Here's the drawing with two shaded views (mm, measured from the low corner). I have some questions. A direction names the side the tool comes from. Coordinates: 2 decimals unless noted, no trailing zeros. Loops run counter-clockwise (first coordinate to the right, second up) from the corner with the lowest first, then second, coordinate; pieces in that order, holes last.
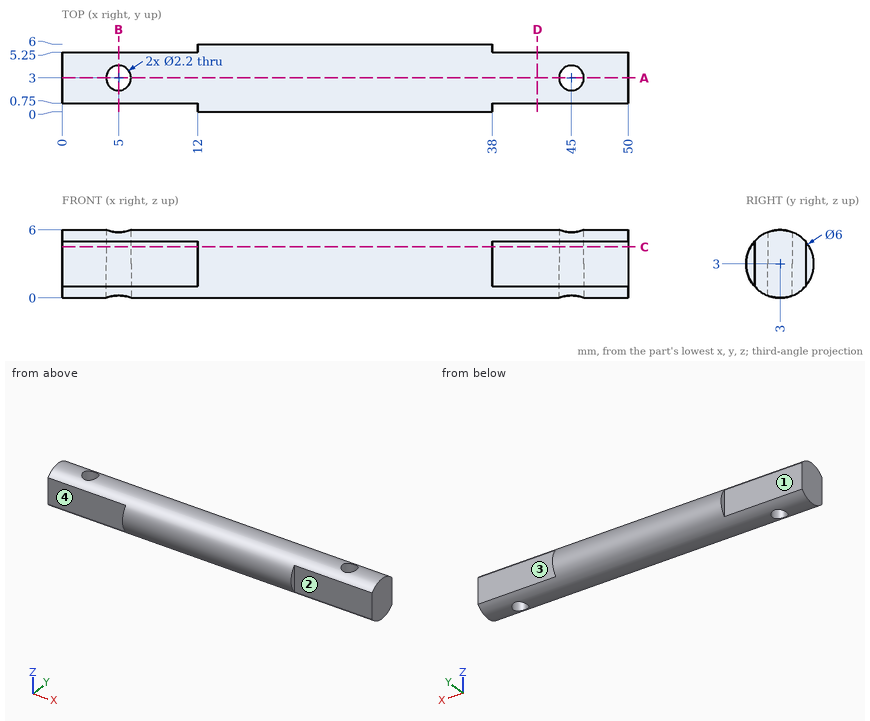
(1) If I drill on probe 1 along Y at (x, z) = (45, 1.15); probe 2 along X at (y, z) = (2, 0.5); probe 3 along X at (y, z) = (2.75, 4.5), over which ranges is the centre line in solid material (lowest first)?
Check values:
probe 1: y = 0.75 to 1.9, 4.1 to 5.25
probe 2: x = 0 to 4.54, 5.46 to 44.54, 45.46 to 50
probe 3: x = 0 to 3.93, 6.07 to 43.93, 46.07 to 50
(2) I want a section at C-C on z = 4.5. Write out the boundary of the cut face in (x, y), then the cut area to 3 significant figures.
Check values:
outline: (0, 0.75) - (12, 0.75) - (12, 0.4) - (38, 0.4) - (38, 0.75) - (50, 0.75) - (50, 5.25) - (38, 5.25) - (38, 5.6) - (12, 5.6) - (12, 5.25) - (0, 5.25) - close; hole circle Ø2.2 at (5, 3); hole circle Ø2.2 at (45, 3)
area: 235 mm2
(3) I'm going to push flat-ended pins straight in: pin 1 (2 mm diameter, centred on x = 41.5, z = 3, fed in from +Y); pin 2 (1.8 mm diameter, centred on x = 5, y = 3, fed in from +Z); pin 3 (1 mm diameter, centred on x = 25, y = 5, fed in from +Z); pin 4 (3 mm diameter, centred on x = 25, y = 5, fed in from -Z). Where does each tip first touch, or does it pass through?
Check values:
pin 1: stops at y = 5.25
pin 2: passes through
pin 3: stops at z = 5.6
pin 4: stops at z = 0.04
(4) I want a section at A-A on y = 3. Write out the boundary of the cut face in (x, z).
Check values:
outline: (0, 0) - (3.9, 0) - (3.9, 6) - (0, 6) - close; (6.1, 0) - (43.9, 0) - (43.9, 6) - (6.1, 6) - close; (46.1, 0) - (50, 0) - (50, 6) - (46.1, 6) - close
(5) I want a section at D-D on x = 42. Write out the boundary of the cut face in (y, z).
Check values:
outline: (0.75, 1.02) arc R3 ccw to (5.25, 1.02) - (5.25, 4.98) arc R3 ccw to (0.75, 4.98) - close
(6) I want a section at B-B on x = 5. Write out the boundary of the cut face in (y, z).
Check values:
outline: (0.75, 1.02) arc R3 ccw to (1.9, 0.21) - (1.9, 5.79) arc R3 ccw to (0.75, 4.98) - close; (4.1, 0.21) arc R3 ccw to (5.25, 1.02) - (5.25, 4.98) arc R3 ccw to (4.1, 5.79) - close
(7) Which directions (+Z, -Z, +X, -X, +Y, -Y) give clear straight access to the entire face, cutting with the end or side of a thin tool? Please do the marked faces 1, 2, 3 and 4.
Check values:
face 1: +Z, -Z, -X, +Y
face 2: +Z, -Z, +X, -Y
face 3: +Z, -Z, +X, +Y
face 4: +Z, -Z, -X, -Y
